Work out the finished part from the listing and answer in its coordinate system (mm). A direction names the side the tool comes from. Coordinates: 2 decimals unless noted, no trailing zeros. Order: outer loops, then holes, each group sorted by start corner. A loop starts at its lowest first (then second) coordinate and runs counter-clockwise, first axis right, second up. Notation, with made-up numbers: M -26.75,-14.75 L 1.25,-14.75 A22 ccw 1.25,21.25 Z; hole C 54.5,45 d1. An arc over 180 degrees is marked long. Answer in a Markdown table with one row per item. Add a question column.
Item 1: Which of the six approach directions +Z, -Z, +X, -X, +Y, -Y give full straight-line access (tool end or side, diameter ignored) to faces 1 (the face through (71, 0, 42.875)), 2 (the face through (-4, 7.938, 30)), 3 (the face through (46, 25.4, 42)), 4 (the face through (22.225, -17, 18))?
Item 2: The part is cut by section A-A (z = 1). Write down the section's boundary in (x, y) (3 decimals).
Item 3: The part is cut by section C-C (x = 77.5). Write down the section's boundary in (y, z), then the cut area to 3 significant figures.
Item 4: Consider line 1 (Z direction, x = -27.5, y = 36) (3 decimals); line 2 (Y direction, x = -23, z = 11.5); line 3 (X direction, y = -14, z = 9) (3 decimals). Determine where each line is inside the solid, lowest interval first. Write a range as from..to.
Item 5: Flat-ended cylindrical pins translate along their axes: pin 1 Ø10 at (x, z) = (38.5, 5) entering from -Y; pin 2 Ø14.5 at (x, y) = (74.5, 8.5) entering from -Z; pin 3 Ø18.5 at (y, z) = (7, 16) entering from +X (3 decimals); pin 4 Ø15.5 at (x, z) = (38, 27) entering from -Y. Find the tip coordinate at first contact, or state that the pin passes through.
Item 6: The part is cut by section D-D (y = 44). Write down the section's boundary in (x, z) (3 decimals).
Item 7: The part is cut by section B-B (y = 22.5). Write down the section's boundary in (x, z) (3 decimals), then the cut area to 3 significant figures.
from build123d import *

# Parameters (mm, degrees)
F1_DEPTH = 63.5
F0_W     = 25.4
F0_H     = 19.05
F2_DEPTH = 25.4
F3_DEPTH = 7.9375
F4_R     = 6.35


with BuildPart() as f1:
    # F0 (on Front) → F1 (new body, symmetric)
    with BuildSketch(Plane.XZ):
        Polygon((41.275, -9.525), (41.275, 9.525), (22.225, 9.525), (-41.275, 9.525), (-41.275, -9.525), align=None)
    extrude(amount=F1_DEPTH, both=True)

    # F0 (on Front) → F2 (join, symmetric)
    with BuildSketch(Plane.XZ):
        with BuildLine():
            Line((22.225, 9.525), (41.275, 9.525))
            Line((41.275, 9.525), (41.275, 27.0002))
            ThreePointArc((41.275, 27.0002), (45.9246798487, 38.2255201513), (57.15, 42.8752))
            Line((57.15, 42.8752), (60.325, 42.8752))
            Line((60.325, 42.8752), (60.325, 61.9252))
            Line((60.325, 61.9252), (57.15, 61.9252))
            ThreePointArc((57.15, 61.9252), (57.0484918683, 61.925052485), (56.9469845941, 61.9246099413))
            ThreePointArc((56.9469845941, 61.9246099413), (32.3826228876, 51.6240229358), (22.225, 27.0002))
            Line((22.225, 27.0002), (22.225, 9.525))
        make_face()
        with Locations((73.025, 52.4002)):
            Rectangle(F0_W, F0_H)
    extrude(amount=F2_DEPTH, both=True)

    # F0 (on Front) → F3 (join, symmetric)
    with BuildSketch(Plane.XZ):
        with BuildLine():
            Line((-41.275, 9.525), (22.225, 9.525))
            Line((22.225, 9.525), (22.225, 27.0002))
            ThreePointArc((22.225, 27.0002), (32.3826228876, 51.6240229358), (56.9469845941, 61.9246099413))
            add(Edge.make_bspline(
                [(-41.275, 9.525), (-40.930863954, 39.584786099), (13.8540179611, 61.7648086868), (56.9469845941, 61.9246099413)],
                knots=[0, 0, 0, 0, 111.3296329326, 111.3296329326, 111.3296329326, 111.3296329326], degree=3))
        make_face()
    extrude(amount=F3_DEPTH, both=True)

    # F4
    f4_edges = [f1.edges().sort_by_distance(p)[0] for p in [
        (-41.275, -63.5, 0),
        (41.275, -63.5, 0),
        (41.275, 63.5, 0),
        (-41.275, 63.5, 0),
    ]]
    fillet(f4_edges, radius=F4_R)


solid = f1.part
Reply:
| question | item | result |
|---|---|---|
| 1 | face 1 | -Z, +X, +Y, -Y |
| 1 | face 2 | +Z, -X, +Y |
| 1 | face 3 | +Z, +X, -X, +Y |
| 1 | face 4 | +Z, -X, -Y |
| 2 | outline | M -41.275,-57.15 A6.35 ccw -34.925,-63.5 L 34.925,-63.5 A6.35 ccw 41.275,-57.15 L 41.275,57.15 A6.35 ccw 34.925,63.5 L -34.925,63.5 A6.35 ccw -41.275,57.15 Z |
| 3 | outline | M -25.4,42.88 L 25.4,42.88 L 25.4,61.93 L -25.4,61.93 Z |
| 3 | area | 968 mm2 |
| 4 | line 1 | z = -9.525..9.525 |
| 4 | line 2 | y = -7.94..7.94 |
| 4 | line 3 | x = -41.275..41.275 |
| 5 | pin 1 | stops at y = -63.5 |
| 5 | pin 2 | stops at z = 42.88 |
| 5 | pin 3 | stops at x = 41.275 |
| 5 | pin 4 | stops at y = -25.4 |
| 6 | outline | M -41.275,-9.525 L 41.275,-9.525 L 41.275,9.525 L -41.275,9.525 Z |
| 7 | outline | M -41.275,-9.525 L 41.275,-9.525 L 41.275,27 A15.875 cw 57.15,42.875 L 85.725,42.875 L 85.725,61.925 L 57.15,61.925 A34.925 ccw 56.947,61.925 A34.925 ccw 22.225,27 L 22.225,9.525 L -41.275,9.525 Z |
| 7 | area | 3,210 mm2 |
